Can you work these out from the drawing? Everything is in mm from the part's minimum corner. Round coordinates to 2 decimals unless told otherwise and drop trailing zeros. Loops run counter-clockwise (first coordinate to the right, second up) from the corner with the lowest first, then second, coordinate; pieces in that order, holes last. Notation, with made-up numbers: M -29.75,66 L 20.25,66 A25 cw 20.25,92 Z; hole C -28,35.5 d6. An arc over 180 degrees is marked long. Use a Markdown table: item, result.
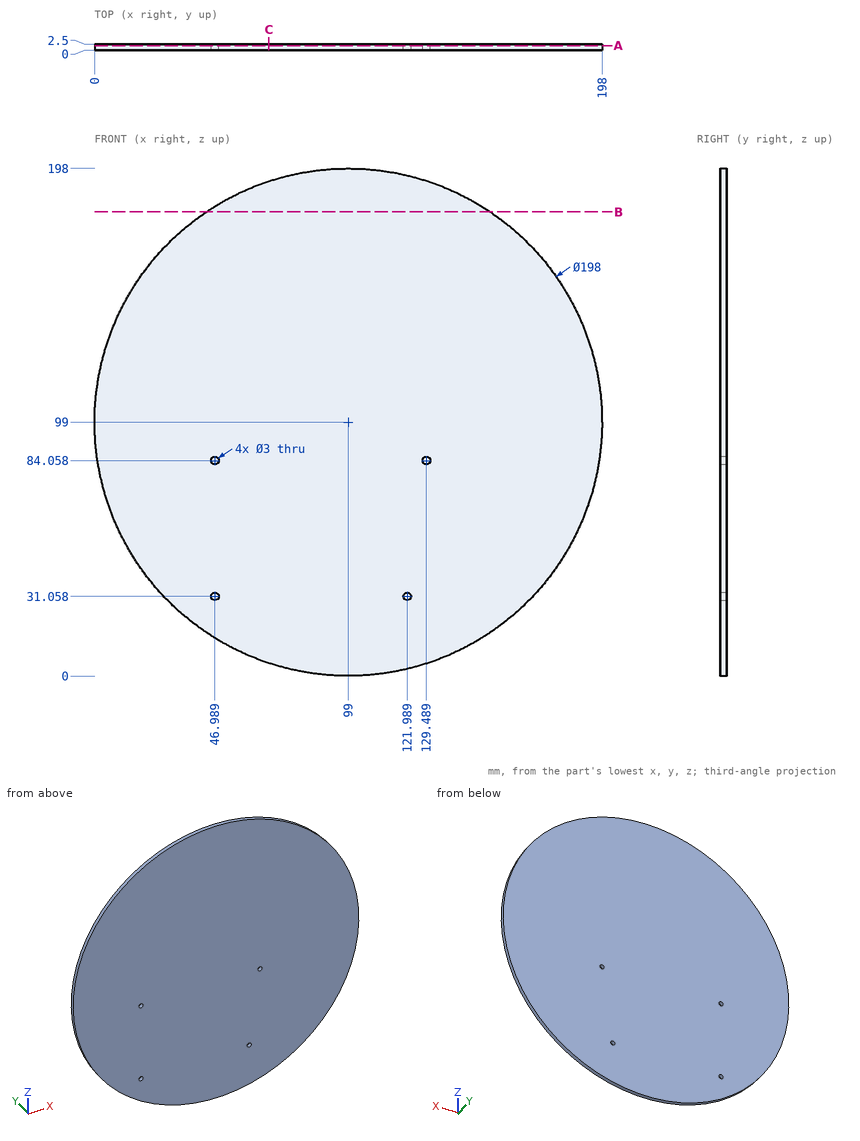
1. Imagine slicing it at C-C, the plane x = 68. Write out the boundary of the cut face in (y, z), then the cut area to 3 significant figures.
Answer sheet:
| item | result |
|---|---|
| outline | M 0,4.98 L 2.5,4.98 L 2.5,193.02 L 0,193.02 Z |
| area | 470 mm2 |
2. Imagine slicing it at B-B, the plane z = 181. Write out the boundary of the cut face in (x, y).
Answer sheet:
| item | result |
|---|---|
| outline | M 43.53,0 L 154.47,0 L 154.47,2.5 L 43.53,2.5 Z |
3. I need wall thicknesses on probe 1 along Z at (x, y) = (86, 1.35); probe 2 along X at (y, z) = (1.6, 72); probe 3 along X at (y, z) = (0.45, 121.5). Which ranges of each line are inside material? Lowest first, please. Write a range as from..to.
Answer sheet:
| item | result |
|---|---|
| probe 1 | 0.86..197.14 |
| probe 2 | 3.75..194.25 |
| probe 3 | 2.59..195.41 |
4. Imagine slicing it at A-A, the plane y = 1.9. Write out the boundary of the cut face in (x, z), then the cut area to 3 significant figures.
Answer sheet:
| item | result |
|---|---|
| outline | C 99,99 d198; hole C 46.99,31.06 d3; hole C 46.99,84.06 d3; hole C 121.99,31.06 d3; hole C 129.49,84.06 d3 |
| area | 30,800 mm2 |
5. For pin 1 Ø1.8 at (x, z) = (46.99, 31.06) entering from +Y; pin 2 Ø1.5 at (x, y) = (153, 1) entering from +Z, each with a flat end and sliding along its axis, tell me the tip position at first contact or that it passes through.
Answer sheet:
| item | result |
|---|---|
| pin 1 | through |
| pin 2 | z = 182.46 |
